Autodesk Inventor part; units mm, degrees
ref_plane "YZ Plane" through (0, 0, 0) normal (1, 0, 0) x (0, 1, 0)
ref_plane "XZ Plane" through (0, 0, 0) normal (0, 1, 0) x (-1, 0, 0)
ref_plane "XY Plane" through (0, 0, 0) normal (0, 0, 1) x (1, 0, 0)
sketch "스케치1" plane through (0, 0, 0) normal (0, 1, 0) x (-1, 0, 0)
  line L0 (12.5, 0) -> (6.25, -10.8253)
  line L1 (6.25, -10.8253) -> (-6.25, -10.8253)
  line L2 (-6.25, -10.8253) -> (-12.5, 0)
  line L3 (-12.5, 0) -> (-6.25, 10.8253)
  line L4 (-6.25, 10.8253) -> (6.25, 10.8253)
  line L5 (6.25, 10.8253) -> (12.5, 0)
  point P0 (0, 0)
  point P1 (0, 0)
  dimension "d0" = 25
extrude "돌출1" add sketch "스케치1" along normal blind 13
sketch "스케치2" plane through (0, 0, 0) normal (0, -1, 0) x (1, 0, 0)
  circle A0 centre (0, 0) radius 8.5
  line L0 (-9, 4.15) -> (9, 4.15)
  line L1 (9, 4.15) -> (9, -4.15)
  line L2 (9, -4.15) -> (-9, -4.15)
  line L3 (-9, -4.15) -> (-9, 4.15)
  line L4 (-9, 4.15) -> (9, -4.15) construction
  line L5 (9, 4.15) -> (-9, -4.15) construction
  point P0 (7.4181, -4.15)
  point P1 (7.4181, 4.15)
  point P2 (-7.4181, -4.15)
  point P3 (-7.4181, 4.15)
  dimension "d3" = 17
  dimension "d4" = 18
  dimension "d5" = 8.3
extrude "돌출2" add sketch "스케치2" along normal blind 25
sketch "스케치3" plane through (0, -25, 0) normal (0, -1, 0) x (1, 0, 0)
  line L0 (8, 0) -> (4, -6.9282)
  line L1 (4, -6.9282) -> (-4, -6.9282)
  line L2 (-4, -6.9282) -> (-8, 0)
  line L3 (-8, 0) -> (-4, 6.9282)
  line L4 (-4, 6.9282) -> (4, 6.9282)
  line L5 (4, 6.9282) -> (8, 0)
  point P0 (0, 0)
  point P1 (0, 0)
  dimension "d8" = 16
extrude "돌출3" add sketch "스케치3" along normal blind 4.5
sketch "스케치4" plane through (0, -29.5, 0) normal (0, -1, 0) x (1, 0, 0)
  arc A0 (-7.4181, -4.15) -> (7.4181, -4.15) centre (0, 0) ccw
  circle A1 centre (0, 0) radius 8.5
  point P0 (7.4181, -4.15)
  dimension "d11" = 17
extrude "돌출4" add sketch "스케치4" along normal blind 40
fillet "모깎기1" radius 0.5 4 edges at (-9, -12.5, 4.15) (9, -12.5, 4.15) (9, -12.5, -4.15) (-9, -12.5, -4.15)
sketch "스케치5" plane through (0, 0, 0) normal (1, 0, 0) x (0, 1, 0)
  line L0 (-8.2, 4) -> (-21.5, 4)
  line L1 (-21.5, 4) -> (-21.5, 13)
  line L2 (-21.5, 13) -> (-8.2, 13)
  line L3 (-8.2, 13) -> (-8.2, 4)
  line L4 (0, 8.5) -> (-25, 8.5) construction
  line L5 (-8.2, 4) -> (-21.5, 13) construction
  line L6 (-21.5, 4) -> (-8.2, 13) construction
  line L7 (-25, 8.5) -> (-25, 4.15)
  line L8 (-12.35, 13) -> (-17.35, 13)
  line L9 (-17.35, 13) -> (-17.35, 4)
  line L10 (-17.35, 4) -> (-12.35, 4)
  line L11 (-12.35, 4) -> (-12.35, 13)
  line L12 (-12.35, 13) -> (-17.35, 4) construction
  line L13 (-17.35, 13) -> (-12.35, 4) construction
  line L14 (-14.85, 13) -> (-14.85, 4)
  line L15 (-8.2, 4) -> (-14.5, 4)
  line L16 (-14.5, 4) -> (-14.5, 4.9729)
  line L17 (-14.5, 4.9729) -> (-8.2, 4.9729)
  line L18 (-8.2, 4.9729) -> (-8.2, 4)
  line L19 (-12.35, 4) -> (-12.35, 4.9729)
  line L20 (-14.5, 4.9729) -> (-17.35, 4.9729)
  line L21 (-17.35, 4.9729) -> (-17.35, 4)
  line L22 (-8.2, 13) -> (-8.2, 10.3)
  line L23 (-8.2, 10.3) -> (-9.2, 4.9729)
  point P0 (0, 0)
  point P1 (-14.85, 8.5)
  point P2 (-14.5, 7.2)
  point P3 (-14.85, 4.9729)
  point P4 (-12.35, 4.9729)
  dimension "d15" = 13.3
  dimension "d17" = 9
  dimension "d18" = 5
  dimension "d31" = 3.5
  dimension "d32" = 2.7
  dimension "d33" = 1
revolve "회전1" add sketch "스케치5" angle 360 about axis through (0, -14.85, 13) along (0, 0, -1) contours L0 L16 L17 L11 | L17 L20 L14 L2 L11 | L11 L2 L3 L23 L17
sketch "스케치8" plane through (0, -14.85, 13) normal (0, 0, 1) x (1, 0, 0)
  circle A0 centre (0, 0) radius 9.55
  line L0 (-9.55, 4.6) -> (9.55, 4.6)
  line L1 (9.55, 4.6) -> (9.55, -4.6)
  line L2 (9.55, -4.6) -> (-9.55, -4.6)
  line L3 (-9.55, -4.6) -> (-9.55, 4.6)
  line L4 (-9.55, 4.6) -> (9.55, -4.6) construction
  line L5 (9.55, 4.6) -> (-9.55, -4.6) construction
  circle A1 centre (0, 0) radius 6.65
  point P0 (0, 14.85)
  point P1 (-4.8023, 4.6)
  point P2 (-8.3691, 4.6)
  point P3 (-8.3691, -4.6)
  point P4 (-4.8023, -4.6)
  point P5 (4.8023, -4.6)
  point P6 (8.3691, -4.6)
  point P7 (8.3691, 4.6)
  point P8 (4.8023, 4.6)
  dimension "d34" = 19.1
  dimension "d35" = 9.2
extrude "돌출7" add sketch "스케치8" against normal blind 1.75 contours A0 L2 A1 L0 | L0 A1 L2 A0 | A1 L2 L0 | L0 A1 | A1 L2
sketch "스케치9" plane through (-8.3691, -10.25, 13) normal (0, 0, 1) x (1, 0, 0)
  arc A0 (13.1715, 0) -> (3.5668, 0) centre (8.3691, -4.6) ccw
  circle A1 centre (8.3691, -4.6) radius 3.65
  line L0 (4.7191, -2.3) -> (12.0191, -2.3)
  line L1 (12.0191, -2.3) -> (12.0191, -6.9)
  line L2 (12.0191, -6.9) -> (4.7191, -6.9)
  line L3 (4.7191, -6.9) -> (4.7191, -2.3)
  line L4 (4.7191, -2.3) -> (12.0191, -6.9) construction
  line L5 (12.0191, -2.3) -> (4.7191, -6.9) construction
  point P0 (8.3691, 10.25)
  point P1 (5.535, -6.9)
  point P2 (11.2033, -6.9)
  point P3 (11.2033, -2.3)
  point P4 (5.535, -2.3)
  dimension "d38" = 7.3
  dimension "d39" = 4.6
extrude "돌출8" add sketch "스케치9" along normal blind 0.2 contours A1 L2 L0 | L0 A1 | A1 L2
extrude "돌출9" add sketch "스케치9" along normal blind 4.1 contours A1 L2 L0
sketch "스케치10" plane through (-8.3691, -10.25, 17.1) normal (0, 0, 1) x (1, 0, 0)
  arc A0 (11.2033, -6.9) -> (11.2033, -2.3) centre (8.3691, -4.6) ccw
  circle A1 centre (8.3691, -4.6) radius 1.5
  point P0 (8.3691, 10.25)
  dimension "d44" = 3
extrude "돌출10" cut sketch "스케치10" against normal blind 4.1
sketch "스케치11" plane through (9, 0, 3.65) normal (1, 0, 0) x (0, 0, -1)
  point P0 (3.65, 0)
properties part number "가스벨브 역설계"
Model file for the job. Use its own axes, mm. A direction names the side the tool comes from. Coordinates: 2 decimals unless noted, no trailing zeros. Order: outer loops, then holes, each group sorted by start corner. A loop starts at its lowest first (then second) coordinate and runs counter-clockwise, first axis right, second up. Notation, with made-up numbers: (-18.75, 70.5) -> (10.25, 70.5) arc R25 cw to (10.25, 83.5) -> close; hole circle Ø5 at (-37, 57). An arc over 180 degrees is marked (long way). Return JSON: item names as keys, results as strings.
Item 1: Pin check, flat tips, straight feed: P1, Ø4, axis at y = -31.5, z = -7.5, coming from the -X side; P2, Ø8, axis at y = -15, z = 0, coming from the -X side; P3, Ø10, axis at x = -0.5, y = -13, coming from the -Z side. Stop position of each tip, or through.
Model answer:
{"P1": "stops at x = -6.48", "P2": "stops at x = -9", "P3": "stops at z = -8.5"}
Item 2: 3-axis set-ups, long thin cutter, end or side, ignore diameter. For faces 4 (the face through (-9, -12, 0)), 5 (the face through (9.55, -14.92, 12.14)), 6 (the face through (0.292, -21.494, 11.331)): which of +Z, -Z, +X, -X, +Y, -Y reach the whole face in a straight line?
Model answer:
{"face 4": "-Z, -X, -Y", "face 5": "+Z, +X", "face 6": "none"}
Item 3: Slice it at A-A (y = -3.5). Write the cut outline in (x, z), then the cut area to 3 significant figures.
Model answer:
{"outline": "(-9, -3.65) arc R0.5 ccw to (-8.5, -4.15) -> (-7.42, -4.15) arc R8.5 ccw to (7.42, -4.15) -> (8.5, -4.15) arc R0.5 ccw to (9, -3.65) -> (9, 3.65) arc R0.5 ccw to (8.5, 4.15) -> (7.42, 4.15) arc R8.5 ccw to (-7.42, 4.15) -> (-8.5, 4.15) arc R0.5 ccw to (-9, 3.65) -> close", "area": "241 mm²"}
Item 4: Slice it at D-D (z = 1.5). Write the cut outline in (x, y).
Model answer:
{"outline": "(-11.63, 0) -> (-9, 0) -> (-9, -25) -> (-7.13, -25) -> (-7.13, -29.5) -> (-8.37, -29.5) -> (-8.37, -69.5) -> (8.37, -69.5) -> (8.37, -29.5) -> (7.13, -29.5) -> (7.13, -25) -> (9, -25) -> (9, 0) -> (11.63, 0) -> (11.63, 13) -> (-11.63, 13) -> close"}
Item 5: Slice it at B-B (z = 9.5). Write the cut outline in (x, y), then the cut area to 3 significant figures.
Model answer:
{"outline": "(-7.02, 0) -> (7.02, 0) -> (7.02, 13) -> (-7.02, 13) -> close; circle Ø13 at (0, -14.85)", "area": "315 mm²"}
Item 6: Mould opens along Y. For faces 1 (the face through (-7, -10.25, 12)), 2 (the face through (0, -27, -6.928)), 3 (the face through (-9.55, -14.78, 12.14)) say: pulls with the +Y half, pulls with the -Y half, needs draft (parallel to the pull), parting line crosses it, or undercut.
Model answer:
{"face 1": "pulls with the +Y half", "face 2": "undercut", "face 3": "parting line crosses it"}
Item 7: Wall check: line 1 along Y through (x, z) = (0, 14.7); line 2 along Y through (x, z) = (0.5, -7.25); line 3 along Z through (x, y) = (6.75, -17). Give the ranges that are in metal, low to high. Write a range as from..to.
Model answer:
{"line 1": "y = -17.15..-16.35, -13.35..-12.55", "line 2": "y = -69.5..-29.5, -25..13", "line 3": "z = -5.17..5.17, 11.25..13"}
